from build123d import *

# Parameters (mm, degrees)
SKETCH2_W           = 44.2
SKETCH2_H           = 44.2
BOSS_EXTRUDE1_DEPTH = 1.5
SKETCH2_3_W         = 44.2
SKETCH2_3_H         = 44.2
SKETCH2_3_W_2       = 41.2
SKETCH2_3_H_2       = 41.2
BOSS_EXTRUDE2_DEPTH = 4.1
SKETCH3_W           = 2.5
SKETCH3_H           = 44.2
BOSS_EXTRUDE3_DEPTH = 1.5
BOSS_EXTRUDE5_DEPTH = 38.2
SKETCH5_W           = 6.546498532
SKETCH5_H           = 41.2
CUT_EXTRUDE1_DEPTH  = 4.1
FILLET2_R           = 0.5


with BuildPart() as part:
    # Sketch2 → Boss-Extrude1 (new body)
    with BuildSketch(Plane(origin=(0, 0, 0), x_dir=(1, 0, 0), z_dir=(0, 1, 0))):
        Rectangle(SKETCH2_W, SKETCH2_H)
    extrude(amount=-BOSS_EXTRUDE1_DEPTH)

    # Sketch2<3> → Boss-Extrude2 (add)
    with BuildSketch(Plane(origin=(0, 0, 0), x_dir=(1, 0, 0), z_dir=(0, 1, 0))):
        Rectangle(SKETCH2_3_W, SKETCH2_3_H)
        Rectangle(SKETCH2_3_W_2, SKETCH2_3_H_2, mode=Mode.SUBTRACT)
    extrude(amount=BOSS_EXTRUDE2_DEPTH)

    # Sketch3 → Boss-Extrude3 (add)
    with BuildSketch(Plane(origin=(0, 4.1, 0), x_dir=(1, 0, 0), z_dir=(0, 1, 0))):
        with Locations((20.85, 0)):
            Rectangle(SKETCH3_W, SKETCH3_H)
    extrude(amount=BOSS_EXTRUDE3_DEPTH)

    # Sketch6 → Boss-Extrude5 (add)
    with BuildSketch(Plane.ZY.offset(-19.6)):
        Polygon((-19.6, 5.6), (-19.6, 4.1), (-20.6, 4.1), (-22.1, 4.1), (-22.1, 5.6), align=None)
        Polygon((19.6, 5.6), (19.6, 4.1), (20.6, 4.1), (22.1, 4.1), (22.1, 5.6), align=None)
    extrude(amount=BOSS_EXTRUDE5_DEPTH)

    # Sketch5 → Cut-Extrude1 (cut)
    with BuildSketch(Plane(origin=(0, 4.1, 0), x_dir=(1, 0, 0), z_dir=(0, 1, 0))):
        with Locations((-23.873249266, 0)):
            Rectangle(SKETCH5_W, SKETCH5_H)
    extrude(amount=-CUT_EXTRUDE1_DEPTH, mode=Mode.SUBTRACT)

    # Fillet2
    fillet2_edges = [part.edges().sort_by_distance(p)[0] for p in [
        (-22.1, 4.1, -21.35),
        (-20.35, 4.1, 22.1),
        (-20.35, 4.1, 20.6),
        (22.1, 5.6, 0),
        (1.75, 5.6, -22.1),
        (1.75, 5.6, 22.1),
        (19.6, 5.6, 0),
        (-20.35, 4.1, -20.6),
        (-20.35, 4.1, -22.1),
        (-18.6, 5.6, -20.85),
        (0.5, 5.6, -19.6),
        (0.5, 5.6, 19.6),
        (-18.6, 5.6, 20.85),
        (-22.1, 1.3, -22.1),
        (-22.1, 1.3, 22.1),
        (22.1, 2.05, 22.1),
        (22.1, 2.05, -22.1),
        (-22.1, 4.1, 21.35),
    ]]
    fillet(fillet2_edges, radius=FILLET2_R)


solid = part.part
Input: part model. Units: mm. Frame: model coordinates. A direction names the side the tool comes from. Coordinates: 2 decimals unless noted, no trailing zeros. Loops run counter-clockwise (first coordinate to the right, second up) from the corner with the lowest first, then second, coordinate; pieces in that order, holes last.
(1) First-contact query: pin 1 Ø8 at (x, z) = (17.5, 7) entering from +Y; pin 2 Ø0.5 at (y, z) = (4.5, -5.5) entering from -X; pin 3 Ø4 at (x, z) = (-9, -16.5) entering from +Y; pin 4 Ø0.6 at (x, z) = (-20.5, -21.5) entering from +Y. Flat tips, straight axial feed; report the tip coordinate or a pass-through.
(2) Section C-C on y = 2.75. Return the cut outline in (x, z), then the cut area to 3 significant figures.
(3) Set-up query: faces 4 (the face through (19.6, 4.6, 0.3)), 5 (the face through (-1, 2, 20.6)), 6 (the face through (22.1, 2, 0)). Return all of +Z, -Z, +X, -X, +Y, -Y with unobstructed straight access to the full face (end or side cutting, diameter ignored); none if empty.
(4) Section A-A on x = -12. Return the cut outline in (y, z).
(5) Pull-direction query (Y, two-part tool) for faces 1 (the face through (-18.6, 4.5, 20.8)), 2 (the face through (20, 4.1, 0)), 3 (the face through (0, -1.5, 0)); classes: released by +Y, released by -Y, zero draft, split by the parting line, or undercut.
(6) Section B-B on z = 10. Return the cut outline in (x, y), then the cut area to 3 significant figures.
(7) Material intervals for probe 1 along Z at (x, y) = (3.5, 2); probe 2 along Z at (x, y) = (7.5, 5); probe 3 along Y at (x, z) = (9, 12), sorted ascending.
Data:
1. pin 1: stops at y = 5.6
1. pin 2: stops at x = 19.6
1. pin 3: stops at y = 0
1. pin 4: stops at y = 4.1
2. outline: (-22.1, -21.6) arc R0.5 ccw to (-21.6, -22.1) - (21.6, -22.1) arc R0.5 ccw to (22.1, -21.6) - (22.1, 21.6) arc R0.5 ccw to (21.6, 22.1) - (-21.6, 22.1) arc R0.5 ccw to (-22.1, 21.6) - (-22.1, 20.6) - (20.6, 20.6) - (20.6, -20.6) - (-22.1, -20.6) - close
2. area: 194 mm2
3. face 4: -X, +Y
3. face 5: -X
3. face 6: +Z, -Z, +X, +Y, -Y
4. outline: (-1.5, -22.1) - (5.1, -22.1) arc R0.5 ccw to (5.6, -21.6) - (5.6, -20.1) arc R0.5 ccw to (5.1, -19.6) - (4.1, -19.6) - (4.1, -20.6) - (0, -20.6) - (0, 20.6) - (4.1, 20.6) - (4.1, 19.6) - (5.1, 19.6) arc R0.5 ccw to (5.6, 20.1) - (5.6, 21.6) arc R0.5 ccw to (5.1, 22.1) - (-1.5, 22.1) - close
5. face 1: zero draft
5. face 2: undercut
5. face 3: released by -Y
6. outline: (-22.1, -1.5) - (22.1, -1.5) - (22.1, 5.1) arc R0.5 ccw to (21.6, 5.6) - (20.1, 5.6) arc R0.5 ccw to (19.6, 5.1) - (19.6, 4.1) - (20.6, 4.1) - (20.6, 0) - (-22.1, 0) - close
6. area: 76.1 mm2
7. probe 1: z = -22.1 to -20.6, 20.6 to 22.1
7. probe 2: z = -22.1 to -19.6, 19.6 to 22.1
7. probe 3: y = -1.5 to 0
